Read the model definition and answer for the solid it produces. Units are mm, in the model's axes. Coordinates: 2 decimals unless noted, no trailing zeros. Order: outer loops, then holes, each group sorted by start corner. A loop starts at its lowest first (then second) coordinate and runs counter-clockwise, first axis right, second up.
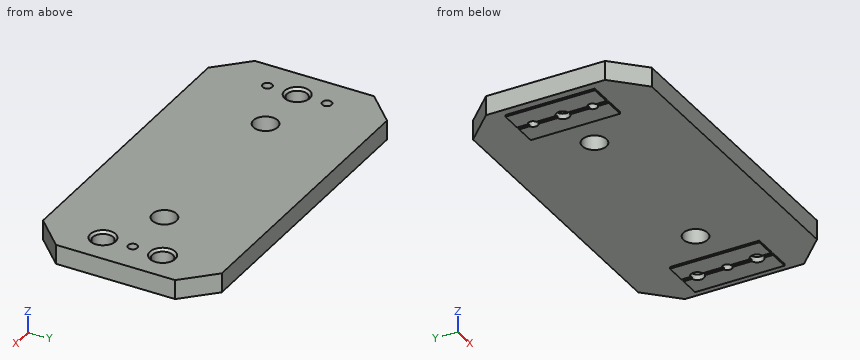
from build123d import *

# Parameters (mm, degrees)
SKETCH1_W                                    = 149.86
SKETCH1_H                                    = 76.2
EXTRUDE1_DEPTH                               = 9.017
SKETCH2_W                                    = 149.86
SKETCH2_H                                    = 76.2
SKETCH2_W_2                                  = 19.05
SKETCH2_H_2                                  = 38.1
CUT_EXTRUDE1_DEPTH                           = 0.762
F_10_32_TAPPED_HOLE1_D                       = 4.0386
CBORE_FOR_10_SOCKET_HEAD_CAP_SCREW1_AT_COUNT = 2
CBORE_FOR_10_SOCKET_HEAD_CAP_SCREW1_AT_PITCH = 124.499845703
CBORE_FOR_10_SOCKET_HEAD_CAP_SCREW1_2_COUNT  = 2
CBORE_FOR_10_SOCKET_HEAD_CAP_SCREW1_2_PITCH  = 25.4
CHAMFER1_SIZE                                = 12.7
SKETCH7_W                                    = 1.5748
SKETCH7_H                                    = 38.1
CUT_EXTRUDE2_DEPTH                           = 0.762
F_13_32_0_40625_DIAMETER_HOLE1_D             = 10.31875


with BuildPart() as part:
    # Sketch1 → Extrude1 (new body)
    with BuildSketch(Plane.XY):
        Rectangle(SKETCH1_W, SKETCH1_H)
    extrude(amount=EXTRUDE1_DEPTH)

    # Sketch2 → Cut-Extrude1 (cut)
    with BuildSketch(Plane(origin=(0, 0, 0), x_dir=(-1, 0, 0), z_dir=(0, 0, -1))):
        Rectangle(SKETCH2_W, SKETCH2_H)
        with Locations((-61.9252, 0)):
            Rectangle(SKETCH2_W_2, SKETCH2_H_2, mode=Mode.SUBTRACT)
        with Locations((61.9252, 0)):
            Rectangle(SKETCH2_W_2, SKETCH2_H_2, mode=Mode.SUBTRACT)
    extrude(amount=-CUT_EXTRUDE1_DEPTH, mode=Mode.SUBTRACT)

    # #10-32 Tapped Hole1 (through all)
    with Locations(Plane.XY.offset(9.017)):
        with Locations((61.9252, 0), (-61.9252, -12.7), (-61.9252, 12.7)):
            Hole(F_10_32_TAPPED_HOLE1_D / 2)

    # Sketch5 → CBORE for #10 Socket Head Cap Screw1 (revolve, cut)
    with BuildSketch(Plane(origin=(61.9252, -12.7, 9.017), x_dir=(0, -1, 0), z_dir=(1, 0, 0))):
        Polygon((0, 0), (0, 9.017), (2.8067, 9.017), (2.8067, 6.6548), (4.3561, 6.6548), (4.3561, 1.0414), (5.3975, 0), align=None)
    cbore_for_10_socket_head_cap_screw1 = revolve(axis=Axis((61.9252, -12.7, 15.367), (0, 0, -1)), mode=Mode.SUBTRACT)

    # CBORE for #10 Socket Head Cap Screw1 at: CBORE for #10 Socket Head Cap Screw1 ×2
    with Locations(*[Vector(-0.994783562, 0.102008159, 0) * (i * CBORE_FOR_10_SOCKET_HEAD_CAP_SCREW1_AT_PITCH) for i in range(1, CBORE_FOR_10_SOCKET_HEAD_CAP_SCREW1_AT_COUNT)]):
        add(cbore_for_10_socket_head_cap_screw1, mode=Mode.SUBTRACT)

    # CBORE for _10 Socket Head Cap Screw1 2: CBORE for #10 Socket Head Cap Screw1 ×2
    with Locations(*[(0, i * CBORE_FOR_10_SOCKET_HEAD_CAP_SCREW1_2_PITCH, 0) for i in range(1, CBORE_FOR_10_SOCKET_HEAD_CAP_SCREW1_2_COUNT)]):
        add(cbore_for_10_socket_head_cap_screw1, mode=Mode.SUBTRACT)

    # Chamfer1
    chamfer1_edges = [part.edges().sort_by_distance(p)[0] for p in [
        (74.93, -38.1, 4.8895),
        (-74.93, -38.1, 4.8895),
        (-74.93, 38.1, 4.8895),
        (74.93, 38.1, 4.8895),
    ]]
    chamfer(chamfer1_edges, length=CHAMFER1_SIZE)

    # Sketch7 → Cut-Extrude2 (cut)
    with BuildSketch(Plane(origin=(0, 0, 0), x_dir=(-1, 0, 0), z_dir=(0, 0, -1))):
        with Locations((61.9252, 0)):
            Rectangle(SKETCH7_W, SKETCH7_H)
        with Locations((-61.9252, 0)):
            Rectangle(SKETCH7_W, SKETCH7_H)
    extrude(amount=-CUT_EXTRUDE2_DEPTH, mode=Mode.SUBTRACT)

    # 13/32 (0.40625) Diameter Hole1 (through all)
    with Locations(Plane.XY.offset(9.017)):
        with Locations((38.1, 0), (-38.1, 0)):
            Hole(F_13_32_0_40625_DIAMETER_HOLE1_D / 2)


solid = part.part
Q1. Straight lines are drawn through the part: L1, parallel to X at y = -12.7, z = 5; L2, parallel to X at y = -12.7, z = 2.25; L3, parallel to Y at x = 38.1, z = 2.5. For each, find the intervals that lie inside material, in ascending order.
Q2. Each of these flat-tipped pins is pushed along its axis until it touches: P1, Ø2.5, axis at x = -61.5, y = 2, coming from the +Z side; P2, Ø1, axis at y = 28, z = 1, coming from the -X side; P3, Ø6, axis at x = 44, y = 24.5, coming from the -Z side; P4, Ø0.8, axis at y = 17, z = 0.5, coming from the +X side. Where does it stop, or does it pass through?
Q3. The part is cut by section C-C, the plane x = 38.1. Determine the outline of the cut face in (y, z).
Q4. The part is cut by section B-B, the plane y = 0. State how many separate pieces and enclosed holes the cut face has, then the cut area to 3 significant figures.
Q5. The part is cut by section A-A, the plane y = 12.7. Determine the outline of the cut face in (x, z).
Computed values:
1. L1: x = -74.93 to -63.94, -59.91 to 57.57, 66.28 to 74.93
1. L2: x = -74.93 to -63.94, -59.91 to 59.12, 64.73 to 74.93
1. L3: y = -38.1 to -5.16, 5.16 to 38.1
2. P1: stops at z = 2.36
2. P2: stops at x = -72.83
2. P3: stops at z = 0.76
2. P4: stops at x = 74.93
3. outline: (-38.1, 0.76) - (-5.16, 0.76) - (-5.16, 9.02) - (-38.1, 9.02) - close; (5.16, 0.76) - (38.1, 0.76) - (38.1, 9.02) - (5.16, 9.02) - close
4. separate pieces: 5
4. enclosed holes: 0
4. area: 987 mm2
5. outline: (-74.93, 0.76) - (-71.45, 0.76) - (-71.45, 0) - (-63.94, 0) - (-63.94, 9.02) - (-74.93, 9.02) - close; (-59.91, 0) - (-52.4, 0) - (-52.4, 0.76) - (52.4, 0.76) - (52.4, 0) - (59.12, 0) - (59.12, 2.36) - (57.57, 2.36) - (57.57, 7.98) - (56.53, 9.02) - (-59.91, 9.02) - close; (64.73, 0) - (71.45, 0) - (71.45, 0.76) - (74.93, 0.76) - (74.93, 9.02) - (67.32, 9.02) - (66.28, 7.98) - (66.28, 2.36) - (64.73, 2.36) - close
